Geometry: final body of the model. Coordinates: model frame, mm. A direction names the side the tool comes from. Give positions to 0.01 mm unless a question says otherwise; leave off trailing zeros. Write each loop counter-clockwise with the first axis right and the second up, starting at its lowest first coordinate (ties: lowest second). Pieces come first, ordered by that corner, then holes. Notation, with made-up numbers: M 54,66 L 97,66 A31 ccw 97,98 Z; hole C 51.5,-18.75 d8. An arc over 180 degrees is marked long. Answer as a JSON object with one key per item and string values.
from build123d import *

# Parameters (mm, degrees)
EXTRUDE_1_DEPTH     = 1.6
EXTRUDE_START       = 1.6
EXTRUDE_2_DEPTH     = 15.2
CUT_EXTRUDE_START   = 35
SKETCH_5_W          = 26.92
SKETCH_5_H          = 1
CUT_EXTRUDE_2_DEPTH = 0.2
CUT_EXTRUDE_START_2 = -35
SKETCH_6_W          = 26.92
SKETCH_6_H          = 1
CUT_EXTRUDE_3_DEPTH = 0.2
CUT_EXTRUDE_START_3 = 16.8
SKETCH_7_W          = 1.6
SKETCH_7_H          = 22.86
SKETCH_7_W_2        = 22.86
SKETCH_7_H_2        = 1.6
CUT_EXTRUDE_4_DEPTH = 9
CUT_EXTRUDE_START_4 = 1.6
SKETCH_8_R          = 1
CUT_EXTRUDE_5_DEPTH = 1.6


with BuildPart() as part:
    # 草图2 → 凸台-拉伸1 (new body)
    with BuildSketch(Plane(origin=(0, 0, 0), x_dir=(1, 0, 0), z_dir=(0, 1, 0))):
        Polygon((-15, 0), (-15, 25), (-35, 25), (-35, 0), (-35, -35), (0, -35), (25, -35), (25, -15), (0, -15), align=None)
    extrude(amount=EXTRUDE_1_DEPTH)

    # 草图3 → 凸台-拉伸2 (add)
    with BuildSketch(Plane(origin=(0, 0, 0), x_dir=(1, 0, 0), z_dir=(0, 1, 0)).offset(EXTRUDE_START)):
        Polygon((-34, -3.46), (-35, -2.46), (-35, 22.46), (-34, 23.46), (-26.8, 23.46), (-25.8, 22.46), (-25.8, -2.46), (-26.8, -3.46), align=None)
        Polygon((22.46, -35), (-2.46, -35), (-3.46, -34), (-3.46, -26.8), (-2.46, -25.8), (22.46, -25.8), (23.46, -26.8), (23.46, -34), align=None)
    extrude(amount=EXTRUDE_2_DEPTH)

    # 草图5 → 切除-拉伸2 (cut)
    with BuildSketch(Plane.XY.offset(CUT_EXTRUDE_START)):
        with Locations((10, 2.1)):
            Rectangle(SKETCH_5_W, SKETCH_5_H)
    extrude(amount=-CUT_EXTRUDE_2_DEPTH, mode=Mode.SUBTRACT)

    # 草图6 → 切除-拉伸3 (cut)
    with BuildSketch(Plane(origin=(0, 0, 0), x_dir=(0, 0, -1), z_dir=(1, 0, 0)).offset(CUT_EXTRUDE_START_2)):
        with Locations((10, 2.1)):
            Rectangle(SKETCH_6_W, SKETCH_6_H)
    extrude(amount=CUT_EXTRUDE_3_DEPTH, mode=Mode.SUBTRACT)

    # 草图7 → 切除-拉伸4 (cut)
    with BuildSketch(Plane(origin=(0, 0, 0), x_dir=(1, 0, 0), z_dir=(0, 1, 0)).offset(CUT_EXTRUDE_START_3)):
        with Locations((-30.4, 10)):
            Rectangle(SKETCH_7_W, SKETCH_7_H)
        with Locations((10, -30.4)):
            Rectangle(SKETCH_7_W_2, SKETCH_7_H_2)
    extrude(amount=-CUT_EXTRUDE_4_DEPTH, mode=Mode.SUBTRACT)

    # 草图8 → 切除-拉伸5 (cut)
    with BuildSketch(Plane(origin=(0, 0, 0), x_dir=(1, 0, 0), z_dir=(0, 1, 0)).offset(CUT_EXTRUDE_START_4)):
        with Locations(Location((-10, -10, 0), (0, 0, 90))):
            Circle(SKETCH_8_R)
    extrude(amount=-CUT_EXTRUDE_5_DEPTH, mode=Mode.SUBTRACT)


solid = part.part
1) Contact query for flat-ended pins moving along their axis: P1, Ø5, axis at y = 6, z = 25, coming from the +X side; P2, Ø1.8, axis at x = -30, z = -5.5, coming from the +Y side; P3, Ø1.8, axis at x = -30.5, y = 13.5, coming from the +Z side; P4, Ø0.5, axis at x = -30.5, y = 14.5, coming from the -Z side. Output: stop coordinate, or through.
Geometry check:
{"P1": "stops at x = 23.46", "P2": "stops at y = 16.8", "P3": "stops at z = 3.46", "P4": "stops at z = -23.46"}
2) Pull-direction query (X, two-part tool) for faces 1 (the flat face through (-3.46, 9, 30)), 2 (the flat face through (10, 7.8, 30)), 3 (the flat face through (-15, 1, -12)); classes: pulls with the +X half, pulls with the -X half, needs draft (parallel to the pull), parting line crosses it, or undercut.
Geometry check:
{"face 1": "pulls with the -X half", "face 2": "undercut", "face 3": "pulls with the +X half"}
3) Line query: line 1 (X direction, y = 11.5, z = -7.5); line 2 (Z direction, x = 7, y = 12); line 3 (Z direction, x = 16, y = 6.25). Output: solid intervals per line, ascending. Write a range as from..to.
Geometry check:
{"line 1": "x = -35..-31.2, -29.6..-25.8", "line 2": "z = 25.8..29.6, 31.2..35", "line 3": "z = 25.8..35"}
4) Set-up query: faces 4 (the flat face through (13, 1, 15)), 5 (the flat face through (-30, 9, 3.46)), 6 (the flat face through (10, 9, 25.8)), 7 (the flat face through (-1.43, 12, 30)), 8 (the flat face through (-25.8, 9, -10)). Return all of +Z, -Z, +X, -X, +Y, -Y with unobstructed straight access to the full face (end or side cutting, diameter ignored); none if empty.
Geometry check:
{"face 4": "-Z, +X, +Y, -Y", "face 5": "+Z, +X, -X, +Y", "face 6": "-Z, +X, -X, +Y", "face 7": "+Y", "face 8": "+Z, -Z, +X, +Y"}
5) Cut plane A-A on y = 10.25. Return loops of the section in (x, z).
Geometry check:
{"outline": "M -35,-22.46 L -34,-23.46 L -26.8,-23.46 L -25.8,-22.46 L -25.8,2.46 L -26.8,3.46 L -34,3.46 L -35,2.46 Z; M -3.46,26.8 L -2.46,25.8 L 22.46,25.8 L 23.46,26.8 L 23.46,34 L 22.46,35 L -2.46,35 L -3.46,34 Z; hole M -31.2,-21.43 L -29.6,-21.43 L -29.6,1.43 L -31.2,1.43 Z; hole M -1.43,29.6 L 21.43,29.6 L 21.43,31.2 L -1.43,31.2 Z"}
6) Cut plane B-B on x = -10. Return loops of the section in (y, z).
Geometry check:
{"outline": "M 0,5 L 1.6,5 L 1.6,9 L 0,9 Z; M 0,11 L 1.6,11 L 1.6,35 L 0,35 Z"}
7) Cut plane D-D on y = 4.25. Return loops of the section in (x, z).
Geometry check:
{"outline": "M -35,-22.46 L -34,-23.46 L -26.8,-23.46 L -25.8,-22.46 L -25.8,2.46 L -26.8,3.46 L -34,3.46 L -35,2.46 Z; M -3.46,26.8 L -2.46,25.8 L 22.46,25.8 L 23.46,26.8 L 23.46,34 L 22.46,35 L -2.46,35 L -3.46,34 Z"}
8) Cut plane C-C on z = 10. Return loops of the section in (x, y).
Geometry check:
{"outline": "M -35,0 L -11,0 L -11,1.6 L -35,1.6 Z; M -9,0 L -5,0 L -5,1.6 L -9,1.6 Z"}
